Geometry: final body of the model. Coordinates: model frame, mm. Face numbers are marked on the shaded views. Give positions to 0.01 mm unless a question says otherwise; leave off trailing zeros. Write each loop counter-clockwise with the first axis right and the second up, starting at its lowest first coordinate (ties: lowest second). Pieces come first, ordered by that corner, then holes. Notation, with made-up numbers: (16, -22) -> (45, -22) arc R10 ccw to (45, -13) -> close; hole circle Ø11 at (-36, 86.25). An arc over 180 degrees is marked (long way). Use CSV: the item, a comma, the result in double quotes. Start each with the question number.
1) Section D-D (y = 190). Output: boundary loops of the cut face in (x, z), plus the area to 3 significant figures.
2) Section B-B (z = 14.5). Count the separate pieces of the cut face and the enclosed holes in it, plus the area to 3 significant figures.
3) Draft query along Y for the marked faces 1, 2 and 3. Return one class per face: pulls with the +Y half, pulls with the -Y half, needs draft (parallel to the pull), parting line crosses it, or undercut.
4) Section A-A (y = 60.5). Output: boundary loops of the cut face in (x, z).
5) Material intervals for line 1 (X direction, y = 57.5, z = 10); line 2 (X direction, y = 67, z = 10.5); line 3 (Y direction, x = -5, z = 13.75), sorted ascending. Write a range as [from, to].
6) Section C-C (x = -13). Output: boundary loops of the cut face in (y, z), plus the area to 3 significant figures.
7) Contact query for flat-ended pins moving along their axis: P1, Ø4, axis at x = 21.5, z = 9.5, coming from the +Y side; P2, Ø10, axis at x = 39.5, z = 16.5, coming from the +Y side; P3, Ø3, axis at y = 157, z = 5, coming from the +X side. Output: stop coordinate, or through.
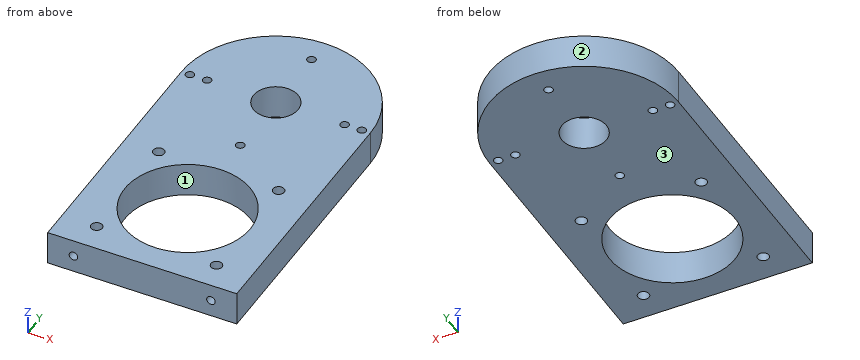
```python
from build123d import *

# Parameters (mm, degrees)
SKETCH1_R                  = 13
BOSS_EXTRUDE1_DEPTH        = 20
F_5_0MM_DOWEL_HOLE1_D      = 5
F_5_0MM_DOWEL_HOLE2_REACH  = 228.164
F_5_0MM_DOWEL_HOLE2_BORE_R = 2.5
F_5_0MM_DOWEL_HOLE3_D      = 5
SKETCH9_R                  = 36.5
CUT_EXTRUDE1_DEPTH         = 214.781968135
F_6_0MM_DOWEL_HOLE1_D      = 6.5


with BuildPart() as part:
    # Sketch1 → Boss-Extrude1 (new body)
    with BuildSketch(Plane.XY):
        with BuildLine():
            Line((-57.251461988, 0), (52.748538012, 0))
            Line((52.748538012, 0), (52.748538012, 150))
            ThreePointArc((52.748538012, 150), (-2.251461988, 205), (-57.251461988, 150))
            Line((-57.251461988, 150), (-57.251461988, 0))
        make_face()
        with Locations((-2.251461988, 150)):
            Circle(SKETCH1_R, mode=Mode.SUBTRACT)
    extrude(amount=BOSS_EXTRUDE1_DEPTH)

    # Ø5.0mm Dowel Hole1 (through all)
    with Locations(Plane(origin=(-2.251461988, 190, 20), x_dir=(1, 0, 0), z_dir=(0, 0, 1))):
        with Locations((0, 0), (40, -40), (0, -80), (-40, -40)):
            Hole(F_5_0MM_DOWEL_HOLE1_D / 2)

    # Ø5.0mm Dowel Hole2 bore (on position points) → Ø5.0mm Dowel Hole2 (cut, up to next)
    with BuildSketch(Plane(origin=(-42.251461988, 0, 10), x_dir=(0, 0, -1), z_dir=(0, -1, 0)), mode=Mode.PRIVATE) as f_5_0mm_dowel_hole2_sk1:
        Circle(F_5_0MM_DOWEL_HOLE2_BORE_R)
    f_5_0mm_dowel_hole2_tool1 = extrude(f_5_0mm_dowel_hole2_sk1.sketch, amount=-F_5_0MM_DOWEL_HOLE2_REACH, mode=Mode.PRIVATE) & part.part
    # Ø5.0mm Dowel Hole2 bore (on position points) → Ø5.0mm Dowel Hole2 (cut, up to next)
    with BuildSketch(Plane(origin=(-42.251461988, 0, 10), x_dir=(0, 0, -1), z_dir=(0, -1, 0)), mode=Mode.PRIVATE) as f_5_0mm_dowel_hole2_sk2:
        with Locations((0, 80)):
            Circle(F_5_0MM_DOWEL_HOLE2_BORE_R)
    f_5_0mm_dowel_hole2_tool2 = extrude(f_5_0mm_dowel_hole2_sk2.sketch, amount=-F_5_0MM_DOWEL_HOLE2_REACH, mode=Mode.PRIVATE) & part.part
    add(f_5_0mm_dowel_hole2_tool1.solids().sort_by_distance((-42.251462, 0, 10))[0], mode=Mode.SUBTRACT)
    add(f_5_0mm_dowel_hole2_tool2.solids().sort_by_distance((37.748538, 0, 10))[0], mode=Mode.SUBTRACT)

    # Ø5.0mm Dowel Hole3 (through all)
    with Locations(Plane(origin=(-52.251461988, 150, 20), x_dir=(1, 0, 0), z_dir=(0, 0, 1))):
        with Locations((0, 0), (100, 0)):
            Hole(F_5_0MM_DOWEL_HOLE3_D / 2)

    # Sketch9 → Cut-Extrude1 (cut, through all)
    with BuildSketch(Plane.XY.offset(20)):
        with Locations((-2.251461988, 51)):
            Circle(SKETCH9_R)
    extrude(amount=-CUT_EXTRUDE1_DEPTH, mode=Mode.SUBTRACT)

    # Ø6.0mm Dowel Hole1 (through all)
    with Locations(Plane(origin=(-37.101461988, 85.85, 20), x_dir=(1, 0, 0), z_dir=(0, 0, 1))):
        with Locations((0, 0), (69.7, 0), (69.7, -69.7), (0, -69.7)):
            Hole(F_6_0MM_DOWEL_HOLE1_D / 2)


solid = part.part
```
Answers follow:
1,outline,"(-40, 0) -> (-4.75, 0) -> (-4.75, 20) -> (-40, 20) -> close; (0.25, 0) -> (35.5, 0) -> (35.5, 20) -> (0.25, 20) -> close"
1,area,"1,410 mm^2"
2,separate pieces,"1"
2,enclosed holes,"12"
2,area,"16,300 mm^2"
3,face 1,"undercut"
3,face 2,"pulls with the +Y half"
3,face 3,"needs draft"
4,outline,"(-57.25, 0) -> (-37.49, 0) -> (-37.49, 20) -> (-57.25, 20) -> close; (32.99, 0) -> (52.75, 0) -> (52.75, 20) -> (32.99, 20) -> close; hole circle Ø5 at (-42.25, 10); hole circle Ø5 at (37.75, 10)"
5,line 1,"x = [-57.25, -44.75], [-39.75, -38.17], [33.67, 35.25], [40.25, 52.75]"
5,line 2,"x = [-57.25, -44.7], [-39.8, -35.06], [30.55, 35.3], [40.2, 52.75]"
5,line 3,"y = [0, 14.6], [87.4, 137.29], [162.71, 204.93]"
6,outline,"(0, 0) -> (16.12, 0) -> (16.12, 20) -> (0, 20) -> close; (85.88, 0) -> (142.69, 0) -> (142.69, 20) -> (85.88, 20) -> close; (157.31, 0) -> (203.94, 0) -> (203.94, 20) -> (157.31, 20) -> close"
6,area,"2,390 mm^2"
7,P1,"stops at y = 200.52"
7,P2,"stops at y = 190.92"
7,P3,"stops at x = 52.47"
